The model under review builds one solid part; all positions refer to its coordinate system, in mm. A direction names the side the tool comes from. Give positions to 0.01 mm unless a question says otherwise; leave off trailing zeros. Order: outer loops, then holes, each group sorted by start corner. A loop starts at its lowest first (then second) coordinate and runs counter-clockwise, first axis right, second up.
Autodesk Inventor part; units mm, degrees
ref_plane "YZ Plane" through (0, 0, 0) normal (1, 0, 0) x (0, 1, 0)
ref_plane "XZ Plane" through (0, 0, 0) normal (0, 1, 0) x (-1, 0, 0)
ref_plane "XY Plane" through (0, 0, 0) normal (0, 0, 1) x (1, 0, 0)
sketch "Sketch1" plane through (0, 0, 0) normal (0, 0, 1) x (1, 0, 0)
  line L0 (0, 0) -> (42.9, 0)
  line L1 (42.9, 0) -> (42.9, 19.7)
  line L2 (42.9, 19.7) -> (0, 19.7)
  line L3 (0, 19.7) -> (0, 0)
  dimension "d0" = 42.9
  dimension "d1" = 19.7
extrude "Extrusion1" add sketch "Sketch1" along normal blind 36
sketch "Sketch2" plane through (0, 0, 36) normal (0, 0, 1) x (1, 0, 0)
  line L0 (3.1975, 17.7737) -> (33.3653, 17.7737)
  line L1 (33.3653, 17.7737) -> (33.3653, 1.0692)
  line L2 (33.3653, 1.0692) -> (3.1975, 1.0692)
  line L3 (3.1975, 1.0692) -> (3.1975, 17.7737)
  point P0 (0, 0)
extrude "Extrusion2" add sketch "Sketch2" along normal blind 3.7
fillet "Fillet1" radius 3 1 edges at (3.1975, 1.0692, 37.85)
fillet "Fillet2" radius 3 1 edges at (3.1975, 17.7737, 37.85)
sketch "Sketch3" plane through (0, 0, 39.7) normal (0, 0, 1) x (1, 0, 0)
  circle A0 centre (9.7525, 9.7525) radius 5
  point P0 (0, 0)
  dimension "d8" = 10
extrude "Extrusion3" add sketch "Sketch3" along normal blind 1
sketch "Sketch4" plane through (9.7525, 9.7525, 40.7) normal (0, 0, 1) x (1, 0, 0)
  circle A0 centre (0, 0) radius 2
  point P0 (-9.7525, -9.7525)
  dimension "d11" = 4
extrude "Extrusion4" add sketch "Sketch4" along normal blind 5
sketch "Sketch5" plane through (0, 0, 0) normal (-1, 0, 0) x (0, 0, 1)
  line L0 (31.9055, 17.6776) -> (29.163, 17.6776)
  line L1 (29.163, 17.6776) -> (29.163, 0.8485)
  line L2 (29.163, 0.8485) -> (31.9055, 0.8485)
  line L3 (31.9055, 0.8485) -> (31.9055, 17.6776)
  point P0 (0, 0)
extrude "Extrusion5" add sketch "Sketch5" along normal blind 7
sketch "Sketch6" plane through (0, 0.8485, 31.9055) normal (0, 0, 1) x (1, 0, 0)
  circle A0 centre (-4.7474, 12.2898) radius 3.3866
  point P0 (0, -0.8485)
extrude "Extrusion6" cut sketch "Sketch6" against normal through all
sketch "Sketch7" plane through (0, 0.8485, 31.9055) normal (0, 0, 1) x (1, 0, 0)
  circle A0 centre (-5.0418, 4.3406) radius 3.2151
  point P0 (0, -0.8485)
extrude "Extrusion7" cut sketch "Sketch7" against normal blind 7
sketch "Sketch8" plane through (42.9, 0, 0) normal (1, 0, 0) x (0, 0, -1)
  line L0 (-31.9055, 1.974) -> (-31.9055, 8.4041)
  line L1 (-31.9055, 1.974) -> (-29.7764, 1.974)
  line L2 (-29.7764, 1.974) -> (-29.7764, 17.7891)
  line L3 (-29.7764, 17.7891) -> (-31.9055, 17.7891)
  line L4 (-31.9055, 17.7891) -> (-31.9055, 1.974)
  point P0 (0, 0)
  point P1 (-31.9055, 7.739)
  point P2 (-31.9055, 2.6391)
extrude "Extrusion8" add sketch "Sketch8" along normal blind 7
sketch "Sketch9" plane through (42.9, 1.974, 31.9055) normal (0, 0, 1) x (1, 0, 0)
  circle A0 centre (4.9018, 3.5919) radius 2.4255
  point P0 (-42.9, -1.974)
extrude "Extrusion9" cut sketch "Sketch9" against normal blind 7
sketch "Sketch10" plane through (42.9, 1.974, 31.9055) normal (0, 0, 1) x (1, 0, 0)
  circle A0 centre (4.6112, 11.0906) radius 3.2917
  point P0 (-42.9, -1.974)
extrude "Extrusion10" cut sketch "Sketch10" against normal blind 7
sketch "Sketch11" plane through (0, 0, 36) normal (0, 0, 1) x (1, 0, 0)
  point P0 (0, 0)
properties part number "sorting"
1. Take a section at C-C (x = 12.5). Write out the cut boundary in (y, z).
2. To check wall thickness, follow line 1 (X direction, y = 15.5, z = 4); line 2 (Z direction, x = 2.5, y = 8); line 3 (Z direction, x = -2, y = 6.75). State the ranges of each line that lie inside material, in increasing order.
3. Take a section at B-B (z = 31). Write out the cut boundary in (x, y), and give its area (3 significant figures).
4. For faces 1 (the flat face through (33.365, 10, 38)), 2 (the cylindrical face through (4.053, 1.971, 37.876)), 3 (the flat face through (46, 1.974, 31)), list the 3-axis set-ups (+Z, -Z, +X, -X, +Y, -Y) from which the entire face can be reached by the end or side of a thin tool; tool diameter is ignored.
5. Insertion check: pin 1 (8 mm diameter, centred on x = 38.5, z = 8, fed in from -Y); pin 2 (11 mm diameter, centred on x = -4.75, y = 13.14, fed in from +Z); pin 3 (0.8 mm diameter, centred on x = -4.5, z = 30, fed in from -Y); pin 4 (3 mm diameter, centred on y = 9, z = 38, fed in from -X). Each pin has a flat end and moves straight along its axis. Give the tip position at first contact, or say it passes through.
6. Take a section at A-A (x = 27.5). Write out the cut boundary in (y, z), and give its area (3 significant figures).
7. Take a section at D-D (z = 16). Write out the cut boundary in (x, y).
Answer:
1. outline: (0, 0) - (19.7, 0) - (19.7, 36) - (17.77, 36) - (17.77, 39.7) - (13.93, 39.7) - (13.93, 40.7) - (5.58, 40.7) - (5.58, 39.7) - (1.07, 39.7) - (1.07, 36) - (0, 36) - close
2. line 1: x = 0 to 42.9
2. line 2: z = 0 to 36
2. line 3: z = 29.16 to 31.91
3. outline: (-7, 0.85) - (0, 0.85) - (0, 0) - (42.9, 0) - (42.9, 1.97) - (49.9, 1.97) - (49.9, 4.35) arc R2.43 cw (long way) to (49.9, 6.78) - (49.9, 10.8) arc R3.29 cw (long way) to (49.9, 15.33) - (49.9, 17.79) - (42.9, 17.79) - (42.9, 19.7) - (0, 19.7) - (0, 17.68) - (-7, 17.68) - (-7, 15.67) arc R3.39 cw (long way) to (-7, 10.61) - (-7, 7.74) arc R3.22 cw (long way) to (-7, 2.64) - close
3. area: 964 mm2
4. face 1: +Z, +X, +Y, -Y
4. face 2: +Z, -X, -Y
4. face 3: +Z, -Z, +X, -Y
5. pin 1: stops at y = 0
5. pin 2: stops at z = 36
5. pin 3: stops at y = 0.85
5. pin 4: stops at x = 3.2
6. outline: (0, 0) - (19.7, 0) - (19.7, 36) - (17.77, 36) - (17.77, 39.7) - (1.07, 39.7) - (1.07, 36) - (0, 36) - close
6. area: 771 mm2
7. outline: (0, 0) - (42.9, 0) - (42.9, 19.7) - (0, 19.7) - close
